Answer from the drawing. Dimensions are ordinates in mm from the lowest x, y and z of the part. Give positions to 0.01 mm unless a question says otherwise; leave off trailing zeros. Write each loop counter-clockwise with the first axis right and the second up, starting at its lowest first coordinate (ties: lowest second). Pieces come first, ordered by that corner, then holes. Notation, with made-up numbers: (-17.75, -8) -> (-9.75, -8) arc R9 cw to (-9.75, 4) -> close; hole circle Ø5 at (28, 61.5). An arc over 180 degrees is marked (long way). Write item = value, one per line.
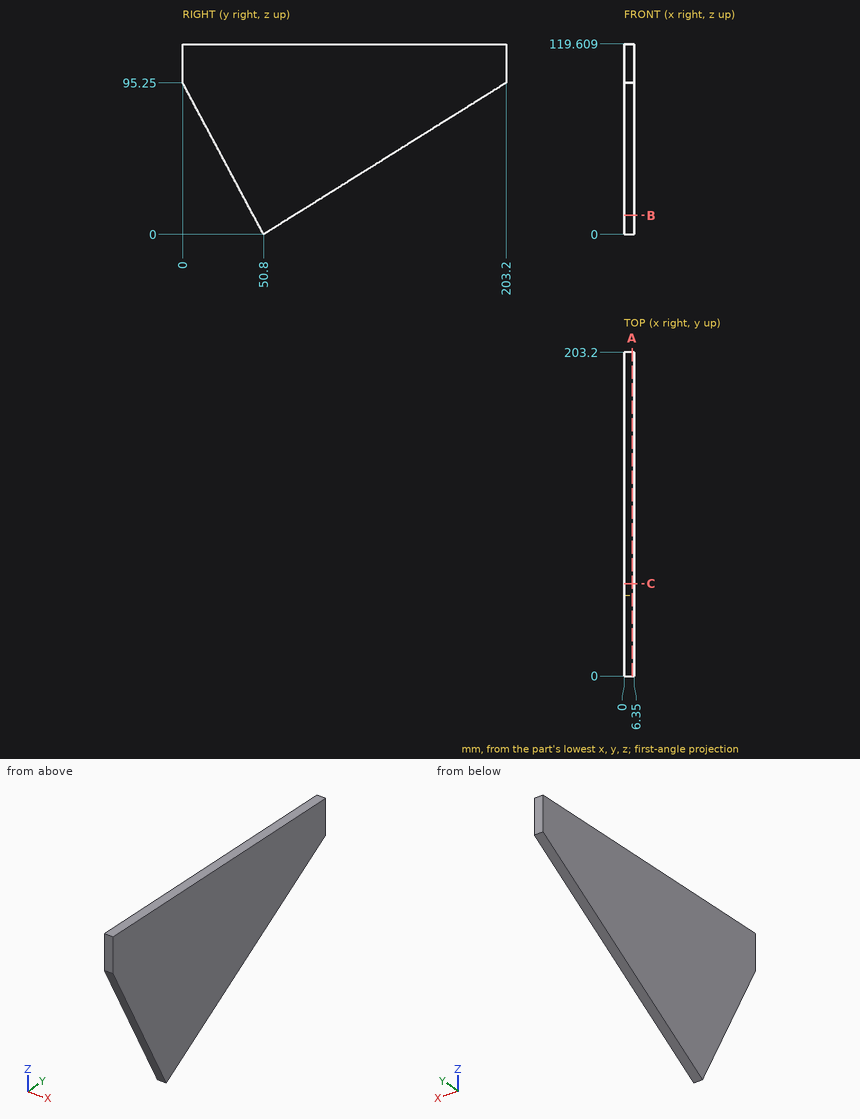
(1) The part is cut by section A-A on x = 5. Determine the outline of the cut face in (y, z), plus the area to 3 significant figures.
Checks:
outline = (0, 95.25) -> (50.8, 0) -> (203.2, 95.25) -> (203.2, 119.61) -> (0, 119.61) -> close
area = 14,600 mm²
(2) The part is cut by section C-C on y = 58. Determine the outline of the cut face in (x, z), plus the area to 3 significant figures.
Checks:
outline = (0, 4.5) -> (6.35, 4.5) -> (6.35, 119.61) -> (0, 119.61) -> close
area = 731 mm²
(3) Consider L1, parallel to Z at x = 3.75, y = 165 (1 decimal); L2, parallel to Z at x = 3.75, y = 28.5 (1 decimal); L3, parallel to Y at x = 1.75, z = 29.5 (1 decimal). Determine where each line is inside the solid, lowest interval first.
Checks:
L1 = 71.4 to 119.6
L2 = 41.8 to 119.6
L3 = 35.1 to 98
(4) The part is cut by section B-B on z = 12. Determine the outline of the cut face in (x, y), plus the area to 3 significant figures.
Checks:
outline = (0, 44.4) -> (6.35, 44.4) -> (6.35, 70) -> (0, 70) -> close
area = 163 mm²
(5) Given P1, Ø1.5, axis at x = 3, y = 162.5, coming from the -Z side, flat-ended and moving along its own axis, determine where the tip first touches the part or whether it passes through.
Checks:
P1 = 69.34
